Can you work these out from the model? Positions are in its coordinate system, mm. A direction names the side the tool comes from. Coordinates: 2 decimals unless noted, no trailing zeros. Write each loop counter-clockwise with the first axis right and the second up, starting at its lowest first coordinate (ties: lowest second). Pieces come first, ordered by that corner, then holes. Notation, with made-up numbers: M 52,-16 L 93,-16 A16 cw 93,14 Z; hole C 34.5,63.5 d11. An arc over 180 degrees is marked long. Use one line per item in the form item = value. Start each with the question number.
Autodesk Inventor part; units mm, degrees
ref_plane "YZ Plane" through (0, 0, 0) normal (1, 0, 0) x (0, 1, 0)
ref_plane "XZ Plane" through (0, 0, 0) normal (0, 1, 0) x (-1, 0, 0)
ref_plane "XY Plane" through (0, 0, 0) normal (0, 0, 1) x (1, 0, 0)
sketch "Sketch1" plane through (0, 0, 0) normal (0, 0, 1) x (1, 0, 0)
  line L0 (-85, 50) -> (85, 50)
  line L1 (85, 50) -> (85, -50)
  line L2 (85, -50) -> (-85, -50)
  line L3 (-85, -50) -> (-85, 50)
  line L4 (-85, 50) -> (85, -50) construction
  line L5 (85, 50) -> (-85, -50) construction
  point P0 (0, 0)
  dimension "d0" = 170
  dimension "d1" = 100
extrude "Extrusion1" add sketch "Sketch1" along normal mid plane 10
sketch "Sketch2" plane through (0, 0, 5) normal (0, 0, 1) x (1, 0, 0)
  line L0 (-70, 35) -> (70, 35)
  line L1 (70, 35) -> (70, -35)
  line L2 (70, -35) -> (-70, -35)
  line L3 (-70, -35) -> (-70, 35)
  line L4 (-70, 35) -> (70, -35) construction
  line L5 (70, 35) -> (-70, -35) construction
  point P0 (0, 0)
  dimension "d4" = 140
  dimension "d5" = 70
extrude "Extrusion2" cut sketch "Sketch2" against normal blind 10
sketch "Sketch3" plane through (0, 0, -5) normal (0, 0, -1) x (-1, 0, 0)
  line L0 (-85, -50) -> (85, -50)
  line L1 (-85, 50) -> (-85, -50)
  line L2 (-85, 50) -> (85, 50)
  point P0 (0, 0)
  point P1 (-27.5, -45)
  point P2 (-80, 25)
  point P3 (-80, -25)
  point P4 (80, 25)
  point P5 (80, -25)
  point P6 (27.5, -45)
  point P7 (-27.5, 45)
  point P8 (27.5, 45)
  dimension "d45" = 5
  dimension "d55" = 50
  dimension "d62" = 160
  dimension "d131" = 25
  dimension "d156" = 57.5
  dimension "d159" = 55
  dimension "d162" = 90
hole "Hole1" at (27.5, -45, -5) at (80, -25, -5) at (80, 25, -5) at (-80, -25, -5) at (-80, 25, -5) at (27.5, 45, -5) at (-27.5, 45, -5) at (-27.5, -45, -5) direction (0, 0, 1) diameter 3.175 depth 5
sketch "Sketch4" plane through (0, 0, 5) normal (0, 0, 1) x (1, 0, 0)
  line L0 (-85, 50) -> (-85, -50)
  line L1 (85, 50) -> (-85, 50)
  line L2 (-85, -50) -> (85, -50)
  line L3 (85, -50) -> (85, 50)
  point P0 (0, 0)
  point P1 (-80, 0)
  point P2 (-80, -45)
  point P3 (0, -45)
  point P4 (-55, -45)
  point P5 (55, -45)
  point P6 (80, -45)
  point P7 (80, 0)
  point P8 (-80, 45)
  point P9 (-55, 45)
  point P10 (55, 45)
  point P11 (0, 45)
  point P12 (80, 45)
  dimension "d3" = 0
  dimension "d72" = 50
  dimension "d73" = 5
  dimension "d74" = 5
  dimension "d75" = 85
  dimension "d78" = 25
  dimension "d80" = 5
  dimension "d81" = 5
  dimension "d82" = 25
  dimension "d85" = 160
  dimension "d115" = 5
  dimension "d116" = 5
  dimension "d117" = 5
  dimension "d120" = 90
  dimension "d125" = 45
hole "Hole2" at (-80, 0, 5) at (-80, -45, 5) at (0, -45, 5) at (-55, -45, 5) at (55, -45, 5) at (80, -45, 5) at (80, 0, 5) at (80, 45, 5) at (55, 45, 5) at (0, 45, 5) at (-55, 45, 5) at (-80, 45, 5) direction (0, 0, -1) diameter 2.5 depth 3
properties part number "top"
1) Which directions (+Z, -Z, +X, -X, +Y, -Y) give clear straight access to the entire face, cutting with the end or side of a thin tool? Please do faces 1 (the face through (-1, -44, -5)), 2 (the face through (-28, -45, 0)), 3 (the face through (-70, 0, 0)).
2) Please list where these lines run through material, in increasing order: line 1 (Y direction, x = 80, z = 3.9); line 2 (X direction, y = 30.5, z = -3.75); line 3 (Y direction, x = -55, z = 2.9).
3) If we mould it in two halves opening along X, with no side actions, what happens to faces 4 (the face through (-80, 25, 0)), 5 (the face through (-1, 50, 0)), 6 (the face through (-85, -1, 0)), 7 (the face through (85, 1, 0))? For each: +X half, -X half, draft (parallel to the pull), parting line (faces both ways), or undercut.
4) Suppose I cut it at C-C on x = -17. Please give me the cut outline in (y, z).
5) Will these pins go through, and if not, where does the flat tip stop? pin 1 Ø2 at (x, y) = (-80, 45) entering from +Z; pin 2 Ø1.6 at (x, y) = (27, -45) entering from -Z; pin 3 Ø4 at (x, y) = (67, 21.5) entering from -Z.
6) Suppose I cut it at B-B on z = -1.5. State how many separate pieces and enclosed holes the cut face has, and give its area (3 significant figures).
7) Suppose I cut it at A-A on y = -5. Please give me the cut outline in (x, z), and give its area (3 significant figures).
Computed values:
q1.face_1 = -Z, +X, -X, +Y, -Y
q1.face_2 = -Z
q1.face_3 = +Z, -Z
q2.line_1 = -50 to -46.25, -43.75 to -1.25, 1.25 to 43.75, 46.25 to 50
q2.line_2 = -85 to -70, 70 to 85
q2.line_3 = -50 to -46.25, -43.75 to -35, 35 to 43.75, 46.25 to 50
q3.face_4 = undercut
q3.face_5 = draft
q3.face_6 = -X half
q3.face_7 = +X half
q4.outline = M -50,-5 L -35,-5 L -35,5 L -50,5 Z; M 35,-5 L 50,-5 L 50,5 L 35,5 Z
q5.pin_1 = 2
q5.pin_2 = 0
q5.pin_3 = through
q6.separate_pieces = 1
q6.enclosed_holes = 9
q6.area = 7,140 mm²
q7.outline = M -85,-5 L -70,-5 L -70,5 L -85,5 Z; M 70,-5 L 85,-5 L 85,5 L 70,5 Z
q7.area = 300 mm²
